Autodesk Inventor part; units mm, degrees
ref_plane "YZ Plane" through (0, 0, 0) normal (1, 0, 0) x (0, 1, 0)
ref_plane "XZ Plane" through (0, 0, 0) normal (0, 1, 0) x (-1, 0, 0)
ref_plane "XY Plane" through (0, 0, 0) normal (0, 0, 1) x (1, 0, 0)
sketch "Sketch1" plane through (0, 0, 0) normal (0, 0, 1) x (1, 0, 0)
  line L0 (-24, 22.8) -> (24, 22.8)
  line L1 (24, 22.8) -> (24, -22.8)
  line L2 (24, -22.8) -> (-24, -22.8)
  line L3 (-24, -22.8) -> (-24, 22.8)
  circle A0 centre (-16, 16.05) radius 2.7
  circle A1 centre (16, 16.05) radius 2.7
  circle A2 centre (16, -15.95) radius 2.7
  circle A3 centre (-16, -15.95) radius 2.7
  line L4 (0, -31.92) -> (0, 31.92)
  line L5 (-33.6, 0) -> (33.6, 0)
  arc A4 (18.7233, 1) -> (1, 18.7233) centre (0, 0) ccw
  arc A5 (-1, 18.7233) -> (-18.7233, 1) centre (0, 0) ccw
  arc A6 (12.9615, 1) -> (1, 12.9615) centre (0, 0) ccw
  arc A7 (-1, 12.9615) -> (-12.9615, 1) centre (0, 0) ccw
  arc A8 (9.933, 1) -> (1, 9.933) centre (0, 0) ccw
  arc A9 (-1, 9.933) -> (-9.933, 1) centre (0, 0) ccw
  arc A10 (-9.9499, -1) -> (-1, -9.9499) centre (0, 0) ccw
  arc A11 (1, -9.933) -> (9.933, -1) centre (0, 0) ccw
  arc A12 (-12.9615, -1) -> (-1, -12.9615) centre (0, 0) ccw
  arc A13 (1, -12.9615) -> (12.9615, -1) centre (0, 0) ccw
  line L6 (-1, -18.7233) -> (-1, -12.9615)
  line L7 (-1, -9.9499) -> (-1, -7.4499)
  line L8 (1, -7.433) -> (1, -9.933)
  line L9 (1, -12.9615) -> (1, -18.7233)
  line L10 (-7.433, 1) -> (-9.933, 1)
  line L11 (-12.9615, 1) -> (-18.7233, 1)
  line L12 (-1, 7.433) -> (-1, 9.933)
  line L13 (-1, 12.9615) -> (-1, 18.7233)
  line L14 (1, 18.7233) -> (1, 12.9615)
  line L15 (1, 9.933) -> (1, 7.433)
  line L16 (18.7233, 1) -> (12.9615, 1)
  line L17 (9.933, 1) -> (7.433, 1)
  line L18 (7.433, -1) -> (9.933, -1)
  line L19 (12.9615, -1) -> (18.7233, -1)
  line L20 (-18.7233, -1) -> (-12.9615, -1)
  line L21 (-9.9499, -1) -> (-7.4499, -1)
  arc A14 (-7.4499, -1) -> (-1, -7.4499) centre (0, 0) ccw
  arc A15 (1, -7.433) -> (7.433, -1) centre (0, 0) ccw
  arc A16 (-1, 7.433) -> (-7.433, 1) centre (0, 0) ccw
  arc A17 (7.433, 1) -> (1, 7.433) centre (0, 0) ccw
  arc A18 (-18.7233, -1) -> (-0.9363, -18.7266) centre (0, 0) ccw
  arc A19 (0.9363, -18.7266) -> (18.7233, -1) centre (0, 0) ccw
  circle A20 centre (16, 16.05) radius 1
  circle A21 centre (-16, 16.05) radius 1
  circle A22 centre (-16, -15.95) radius 1
  circle A23 centre (16, -15.95) radius 1
  point P0 (-24, 0)
  point P1 (-24, 0)
  point P2 (0, 22.8)
  point P3 (0, 22.8)
  dimension "d4" = 48
  dimension "d5" = 45.6
  dimension "d6" = 5.4
  dimension "d7" = 5.4
  dimension "d8" = 5.4
  dimension "d9" = 5.4
  dimension "d10" = 16
  dimension "d11" = 16
  dimension "d12" = 15.95
  dimension "d13" = 16.05
  dimension "d22" = 2.5
  dimension "d28" = 2
  dimension "d29" = 2
  dimension "d30" = 2
  dimension "d31" = 2
extrude "Extrusion1" add sketch "Sketch1" along normal blind 0.8 contours L0 L4 L5 L3 | L0 L1 L5 L4 | L5 L4 L2 L3 | L5 L1 L2 L4 | A0 | A1 | A2 | A3 | A20 | A21 | A22 | A23
sketch "Sketch2" plane through (0, 0, 0) normal (0, 0, -1) x (-1, 0, 0)
  line L0 (-24, 22.8) -> (24, 22.8)
  line L1 (-24, -22.8) -> (-24, 22.8)
  line L2 (24, -22.8) -> (-24, -22.8)
  line L3 (24, 22.8) -> (24, -22.8)
  line L4 (23.2, 22) -> (-23.2, 22)
  line L5 (-23.2, 22) -> (-23.2, -22)
  line L6 (-23.2, -22) -> (23.2, -22)
  line L7 (23.2, -22) -> (23.2, 22)
  point P0 (0, 0)
  dimension "d25" = 0.8
extrude "Extrusion2" add sketch "Sketch2" along normal blind 42
sketch "Sketch3" plane through (0, 0, 0) normal (0, 0, -1) x (-1, 0, 0)
  circle A0 centre (-16, 16.05) radius 2.7
  circle A1 centre (16, 16.05) radius 2.7
  circle A2 centre (16, -15.95) radius 2.7
  circle A3 centre (-16, -15.95) radius 2.7
  line L0 (33.6, 0) -> (-33.6, 0)
  line L1 (0, -31.92) -> (0, 31.92)
  point P0 (0, 0)
  dimension "d32" = 5.4
  dimension "d33" = 5.4
  dimension "d34" = 5.4
  dimension "d35" = 5.4
  dimension "d36" = 16.05
  dimension "d37" = 15.95
  dimension "d38" = 16
  dimension "d39" = 16
extrude "Extrusion3" add sketch "Sketch3" along normal blind 4.2
sketch "Sketch4" plane through (16, 16.05, -4.2) normal (0, 0, -1) x (-1, 0, 0)
  circle A0 centre (0, 0) radius 2.7
  circle A1 centre (32, 0) radius 2.7
  circle A2 centre (32, -32) radius 2.7
  circle A3 centre (0, -32) radius 2.7
  point P0 (16, -16.05)
hole "Hole1" at (16, 16.05, -4.2) at (-16, 16.05, -4.2) at (-16, -15.95, -4.2) at (16, -15.95, -4.2) direction (0, 0, 1) diameter 2.459 depth 4
sketch "Sketch5" plane through (-24, 22.8, 0.8) normal (0, 1, 0) x (1, 0, 0)
  line L0 (0, 42.8) -> (48, 42.8)
  line L1 (48, 42.8) -> (21.8, 42.8)
  line L2 (0.8, 42.8) -> (47.2, 42.8)
  line L3 (47.2, 22.8) -> (21, 22.8)
  line L4 (21, 22.8) -> (21, 42.8)
  line L5 (21, 42.8) -> (47.2, 42.8)
  line L6 (47.2, 42.8) -> (47.2, 22.8)
  line L7 (48, 0) -> (48, 42.8)
  point P0 (24, 0.8)
  dimension "d53" = 26.2
  dimension "d54" = 20
  dimension "d55" = 0.8
extrude "Extrusion4" cut sketch "Sketch5" against normal up to surface (0.8 mm away)
sketch "Sketch6" plane through (-23.2, -22, 0) normal (0, 1, 0) x (1, 0, 0)
  line L0 (47.2, 42) -> (-0.8, 42)
  line L1 (46.4, 42) -> (8.2, 42)
  line L2 (8.2, 42) -> (8.2, 11)
  line L3 (8.2, 11) -> (46.4, 11)
  line L4 (46.4, 11) -> (46.4, 42)
  line L5 (47.2, 42) -> (47.2, -0.8)
  point P0 (23.2, 0)
  dimension "d56" = 0.8
  dimension "d57" = 38.2
  dimension "d58" = 31
extrude "Extrusion5" cut sketch "Sketch6" against normal up to surface (0.8 mm away)
fillet "Fillet1" radius 2 2 edges at (-3, 22.4, -22) (-15, -22.4, -11)
sketch "Sketch7" plane through (-24, -22.8, 0.8) normal (-1, 0, 0) x (0, 0, 1)
  line L0 (-38.3, 37.6) -> (-13.3, 37.6) construction
  line L1 (-38.3, 36.1) -> (-13.3, 36.1)
  line L2 (-13.3, 39.1) -> (-38.3, 39.1)
  arc A0 (-38.3, 39.1) -> (-38.3, 36.1) centre (-38.3, 37.6) ccw
  arc A1 (-13.3, 36.1) -> (-13.3, 39.1) centre (-13.3, 37.6) ccw
  line L3 (-42.8, 45.6) -> (0, 45.6)
  line L4 (-42.8, 0) -> (-42.8, 45.6)
  line L5 (-13.3, 34.1) -> (-38.3, 34.1)
  arc A2 (-38.3, 34.1) -> (-38.3, 31.1) centre (-38.3, 32.6) ccw
  line L6 (-38.3, 31.1) -> (-13.3, 31.1)
  arc A3 (-13.3, 31.1) -> (-13.3, 34.1) centre (-13.3, 32.6) ccw
  line L7 (-13.3, 29.1) -> (-38.3, 29.1)
  arc A4 (-38.3, 29.1) -> (-38.3, 26.1) centre (-38.3, 27.6) ccw
  line L8 (-38.3, 26.1) -> (-13.3, 26.1)
  arc A5 (-13.3, 26.1) -> (-13.3, 29.1) centre (-13.3, 27.6) ccw
  point P0 (-0.8, 22.8)
  point P1 (-25.8, 37.6)
  dimension "d63" = 3
  dimension "d64" = 25
  dimension "d65" = 8
  dimension "d66" = 17
  dimension "d69" = 5
extrude "Extrusion6" cut sketch "Sketch7" against normal up to surface (0.8 mm away)
sketch "Sketch8" plane through (24, -22.8, 0.8) normal (1, 0, 0) x (0, 0, -1)
  line L0 (0, 45.6) -> (42.8, 45.6)
  line L1 (42.8, 45.6) -> (42.8, 0)
  point P0 (0.8, 22.8)
  point P1 (2.8, 41)
  point P2 (37.8, 41)
  point P3 (37.8, 6)
  point P4 (2.8, 6)
  dimension "d76" = 4.6
  dimension "d77" = 39.6
  dimension "d78" = 40
  dimension "d79" = 5
hole "Hole2" at (24, 18.2, -2) at (24, 18.2, -37) at (24, -16.8, -37) at (24, -16.8, -2) direction (-1, 0, 0) diameter 1.567 depth 4.55
sketch "Sketch9" plane through (0, 0, -42) normal (0, 0, -1) x (-1, 0, 0)
  line L0 (-24, -22.8) -> (-24, 22.8)
  line L1 (24, -22.8) -> (-24, -22.8)
  line L2 (-24, 22.8) -> (-23.2, 22.8)
  line L3 (-23.2, 22.8) -> (-23.2, -22.8)
  line L4 (-23.2, -22.8) -> (-24, -22.8)
  line L5 (-24, -22.8) -> (-24, 22.8)
  point P0 (0, 0)
  dimension "d87" = 0.8
extrude "Extrusion7" add sketch "Sketch9" along normal blind 2.8
sketch "Sketch10" plane through (24, -22.8, 0.8) normal (1, 0, 0) x (0, 0, -1)
  line L0 (45.6, 0) -> (45.6, 45.6)
  line L1 (45.6, 0) -> (11.8, 0)
  line L2 (11.8, 0) -> (11.8, 2)
  line L3 (11.8, 2) -> (45.6, 2)
  line L4 (45.6, 2) -> (45.6, 0)
  point P0 (0.8, 22.8)
  point P1 (45.6, 2)
  dimension "d90" = 33.8
  dimension "d91" = 2
extrude "Extrusion8" cut sketch "Sketch10" against normal up to surface (0.8 mm away)
sketch "Sketch11" plane through (0, 0, -42) normal (0, 0, -1) x (-1, 0, 0)
  circle A0 centre (10.5, 27.25) radius 2
  circle A1 centre (28, 8.35) radius 2
  line L0 (24, 22.8) -> (3, 22.8)
  arc A2 (15.75, 27.25) -> (5.25, 27.25) centre (10.5, 27.25) ccw
  line L1 (23.2, 22) -> (-23.2, 22)
  line L2 (5.25, 27.25) -> (5.25, 22.8)
  line L3 (15.75, 27.25) -> (15.75, 22.8)
  arc A3 (28, 4.35) -> (28, 12.35) centre (28, 8.35) ccw
  line L4 (28, 12.35) -> (24, 12.35)
  line L5 (24, 22.8) -> (24, -22.8)
  line L6 (28, 4.35) -> (24, 4.35)
  point P0 (0, 0)
  point P1 (10.5, 31.85)
  dimension "d94" = 4
  dimension "d95" = 4
  dimension "d96" = 28
  dimension "d97" = 27.25
  dimension "d98" = 10.5
  dimension "d99" = 8.35
  dimension "d100" = 31.85
  dimension "d101" = 8
extrude "Extrusion9" add sketch "Sketch11" against normal blind 0.8
properties part number "Fan Cover" material "Aluminum 6061"
Model file for the job. Use its own axes, mm. A direction names the side the tool comes from. Give positions to 0.01 mm unless a question says otherwise; leave off trailing zeros. Loops run counter-clockwise (first coordinate to the right, second up) from the corner with the lowest first, then second, coordinate; pieces in that order, holes last. Notation, with made-up numbers: (67.5, -1.5) -> (119.5, -1.5) arc R7 cw to (119.5, 5.5) -> close; hole circle Ø9 at (-4, 22.5). An arc over 180 degrees is marked (long way). Write each question's results on one line, items separated by ' | '.
(1) Pull direction Z, two halves, no side cores. Call faces 4 (the flat face through (-26, 10, -41.2)), 5 (the cylindrical face through (-23.6, 9.8, -39)), 6 (the cylindrical face through (-23.6, 9.8, -11)), 7 (the cylindrical face through (-10.6, 32.5, -41.6)): released by +Z, released by -Z, zero draft, split by the parting line, or undercut.
Geometry results:
face 4: released by +Z | face 5: undercut | face 6: undercut | face 7: zero draft
(2) Cut at C-C on y = 26. List the corners of the cut face in (x, z), and give its area (3 significant figures).
Geometry results:
outline: (-15.75, -42) -> (-12.06, -42) -> (-12.06, -41.2) -> (-15.75, -41.2) -> close; (-8.94, -42) -> (-5.25, -42) -> (-5.25, -41.2) -> (-8.94, -41.2) -> close | area: 5.90 mm²
(3) Flat gauge pins, fed straight in: pin 1 Ø8 at (x, y) = (-3, 23) entering from -Z; pin 2 Ø6 at (x, y) = (-5.5, -15) entering from -Z; pin 3 Ø2.5 at (x, y) = (15, 15) entering from -Z; pin 4 Ø1 at (x, y) = (16.5, 2) entering from +Z. Where does each tip first touch, or does it go through?
Geometry results:
pin 1: stops at z = -42 | pin 2: stops at z = 0 | pin 3: stops at z = -4.2 | pin 4: passes through
(4) Cut at B-B on z = -18.5. List the corners of the cut face in (x, y).
Geometry results:
outline: (-24, -22.8) -> (-15, -22.8) -> (-15, -22) -> (-23.2, -22) -> (-23.2, 3.3) -> (-24, 3.3) -> close; (-24, 6.3) -> (-23.2, 6.3) -> (-23.2, 8.3) -> (-24, 8.3) -> close; (-24, 11.3) -> (-23.2, 11.3) -> (-23.2, 13.3) -> (-24, 13.3) -> close; (-24, 16.3) -> (-23.2, 16.3) -> (-23.2, 22) -> (23.2, 22) -> (23.2, -20.8) -> (24, -20.8) -> (24, 22.8) -> (-24, 22.8) -> close
(5) Tool access for faces 1 (the cylindrical face through (-5.351, 5.255, 0.394)), 2 (the cylindrical face through (-23.6, 4.8, -11)), 3 (the flat face through (-16, -16, -0.2)): list every direction of +Z, -Z, +X, -X, +Y, -Y with a clear straight run to the whole face (end or side of a thin tool).
Geometry results:
face 1: +Z, -Z | face 2: -X | face 3: -Z
(6) Probe line 1 along Y through (x, z) = (16, -1.55); line 2 along Y through (x, z) = (-10.5, -41.8); line 3 along Y through (x, z) = (-28, -41.75). List the from-to ranges inside material, lowest first.
Geometry results:
line 1: y = -22.8 to -22, -18.65 to -17.18, -14.72 to -13.25, 13.35 to 14.82, 17.28 to 18.75, 22 to 22.8 | line 2: y = 22 to 25.25, 29.25 to 32.5 | line 3: y = 4.35 to 6.35, 10.35 to 12.35
(7) Cut at A-A on z = -2. Give the number of separate pieces and of enclosed holes in the cut face, and give its area (3 significant figures).
Geometry results:
separate pieces: 6 | enclosed holes: 4 | area: 217 mm²
(8) Cut at D-D on x = 2.5. List the corners of the cut face in (y, z), and give its area (3 significant figures).
Geometry results:
outline: (-22.8, -11) -> (-22, -11) -> (-22, 0) -> (-18.58, 0) -> (-18.58, 0.8) -> (-22.8, 0.8) -> close; (-12.76, 0) -> (-9.67, 0) -> (-9.67, 0.8) -> (-12.76, 0.8) -> close; (-7.07, 0) -> (7.07, 0) -> (7.07, 0.8) -> (-7.07, 0.8) -> close; (9.67, 0) -> (12.76, 0) -> (12.76, 0.8) -> (9.67, 0.8) -> close; (18.58, 0) -> (22, 0) -> (22, -22) -> (22.8, -22) -> (22.8, 0.8) -> (18.58, 0.8) -> close | area: 49.4 mm²
